Autodesk Inventor part; units mm, degrees
ref_plane "YZ Plane" through (0, 0, 0) normal (1, 0, 0) x (0, 1, 0)
ref_plane "XZ Plane" through (0, 0, 0) normal (0, 1, 0) x (-1, 0, 0)
ref_plane "XY Plane" through (0, 0, 0) normal (0, 0, 1) x (1, 0, 0)
sketch "Sketch1" plane through (0, 0, 0) normal (0, 0, 1) x (1, 0, 0)
  line L0 (-30, 25) -> (30, 25)
  line L1 (30, 25) -> (30, -25)
  line L2 (30, -25) -> (-30, -25)
  line L3 (-30, -25) -> (-30, 25)
  point P0 (0, 0)
  point P1 (30, 0)
  point P2 (0, 25)
  dimension "d0" = 60
  dimension "d1" = 50
extrude "Extrusion1" add sketch "Sketch1" along normal blind 2
fillet "Fillet1" radius 2 4 edges at (30, 25, 1) (-30, 25, 1) (30, -25, 1) (-30, -25, 1)
sketch "Sketch2" plane through (0, 0, 2) normal (0, 0, 1) x (1, 0, 0)
  line L0 (-25, 20) -> (25, 20) construction
  line L1 (25, 20) -> (25, -20) construction
  line L2 (25, -20) -> (-25, -20) construction
  line L3 (-25, -20) -> (-25, 20) construction
  point P0 (0, 0)
  point P1 (25, 0)
  point P2 (0, 20)
  dimension "d5" = 50
  dimension "d6" = 40
hole "Hole1" at (-25, 20, 2) at (25, 20, 2) at (-25, -20, 2) at (25, -20, 2) direction (0, 0, -1) diameter 3.4 end through all
sketch "Sketch3" plane through (0, 0, 2) normal (0, 0, 1) x (1, 0, 0)
  line L0 (-18.5, 19) -> (18.5, 19)
  line L1 (18.5, 19) -> (18.5, -14)
  line L2 (18.5, -14) -> (-18.5, -14)
  line L3 (-18.5, -14) -> (-18.5, 19)
  point P0 (0, 0)
  point P1 (0, 19)
  dimension "d15" = 33
  dimension "d16" = 37
  dimension "d17" = 14
extrude "Extrusion2" cut sketch "Sketch3" against normal blind 2
fillet "Fillet2" radius 2 4 edges at (-18.5, 19, 1) (18.5, 19, 1) (18.5, -14, 1) (-18.5, -14, 1)
sketch "Sketch4" plane through (0, 0, 2) normal (0, 0, 1) x (1, 0, 0)
  line L0 (-6.75, -17.5) -> (14.75, -17.5) construction
  line L1 (16.5, -14) -> (-16.5, -14)
  point P0 (0, 0)
  point P1 (4, -17.5)
  dimension "d21" = 21.5
  dimension "d22" = 3.5
  dimension "d33" = 4
hole "Hole2" at (-6.75, -17.5, 2) at (14.75, -17.5, 2) direction (0, 0, -1) diameter 3.4 end through all
chamfer "Chamfer1" distance 0.4 angle 45 44 edges at (0, 25, 2) (-29.4142, 24.4142, 2) (-30, 0, 2) (-29.4142, -24.4142, 2) (0, -25, 2) (29.4142, -24.4142, 2) (30, 0, 2) (29.4142, 24.4142, 2) (0, 25, 0) (-29.4142, 24.4142, 0) (-30, 0, 0) (-29.4142, -24.4142, 0) (0, -25, 0) (29.4142, -24.4142, 0) (30, 0, 0) (29.4142, 24.4142, 0) (-18.5, 2.5, 0) (-17.9142, -13.4142, 0) (0, -14, 0) (17.9142, -13.4142, 0) (18.5, 2.5, 0) (17.9142, 18.4142, 0) (0, 19, 0) (-17.9142, 18.4142, 0) (0, 19, 2) (17.9142, 18.4142, 2) (18.5, 2.5, 2) (17.9142, -13.4142, 2) (0, -14, 2) (-17.9142, -13.4142, 2) (-18.5, 2.5, 2) (-17.9142, 18.4142, 2) (-25, -18.3, 2) (25, -18.3, 2) (-25, 21.7, 2) (25, 21.7, 2) (-6.75, -15.8, 2) (14.75, -15.8, 2) (-25, -18.3, 0) (25, -18.3, 0) (-25, 21.7, 0) (25, 21.7, 0) (-6.75, -15.8, 0) (14.75, -15.8, 0)
properties part number "bradboardclip" material "ABS Plastic"
Build history of the part. All positions in model axes, mm. A direction names the side the tool comes from. Give positions to 0.01 mm unless a question says otherwise; leave off trailing zeros. Loops run counter-clockwise (first coordinate to the right, second up) from the corner with the lowest first, then second, coordinate; pieces in that order, holes last. Notation, with made-up numbers: (17.25, 33) - (75.25, 33) arc R12 cw to (75.25, 48) - close; hole circle Ø8 at (6, 49). An arc over 180 degrees is marked (long way). Use a Markdown table: item, result.
(1) Wall check: line 1 along X through (y, z) = (20, 1.4); line 2 along Y through (x, z) = (25, 1.05); line 3 along X through (y, z) = (-17.5, 0.85). Give the ranges that are in metal, low to high.
Taken from the geometry:
| item | result |
|---|---|
| line 1 | -30 to -26.7, -23.3 to 23.3, 26.7 to 30 |
| line 2 | -25 to -21.7, -18.3 to 18.3, 21.7 to 25 |
| line 3 | -30 to -8.45, -5.05 to 13.05, 16.45 to 30 |
(2) Band-saw the part on C-C (y = 14). Give the cut face in (x, z), and give its area (3 significant figures).
Taken from the geometry:
| item | result |
|---|---|
| outline | (-30, 0.4) - (-29.6, 0) - (-18.9, 0) - (-18.5, 0.4) - (-18.5, 1.6) - (-18.9, 2) - (-29.6, 2) - (-30, 1.6) - close; (18.5, 0.4) - (18.9, 0) - (29.6, 0) - (30, 0.4) - (30, 1.6) - (29.6, 2) - (18.9, 2) - (18.5, 1.6) - close |
| area | 45.4 mm2 |
(3) Drop flat-ended pins along their axis: pin 1 Ø3 at (x, y) = (-25, -20) entering from -Z; pin 2 Ø4 at (x, y) = (25, -20) entering from +Z; pin 3 Ø4 at (x, y) = (-25, 20) entering from -Z. Give the stop position or say it passes through.
Taken from the geometry:
| item | result |
|---|---|
| pin 1 | through |
| pin 2 | z = 1.9 |
| pin 3 | z = 0.1 |
(4) Band-saw the part on B-B (x = 25). Give the cut face in (y, z), and give its area (3 significant figures).
Taken from the geometry:
| item | result |
|---|---|
| outline | (-25, 0.4) - (-24.6, 0) - (-22.1, 0) - (-21.7, 0.4) - (-21.7, 1.6) - (-22.1, 2) - (-24.6, 2) - (-25, 1.6) - close; (-18.3, 0.4) - (-17.9, 0) - (17.9, 0) - (18.3, 0.4) - (18.3, 1.6) - (17.9, 2) - (-17.9, 2) - (-18.3, 1.6) - close; (21.7, 0.4) - (22.1, 0) - (24.6, 0) - (25, 0.4) - (25, 1.6) - (24.6, 2) - (22.1, 2) - (21.7, 1.6) - close |
| area | 85.4 mm2 |
(5) Pull direction Y, two halves, no side cores. Call faces 1 (the face through (0, -25, 1)), 2 (the face through (30, 0, 1)), 3 (the face through (17.978, 18.511, 0.286)), 4 (the face through (-17.978, 18.511, 1.714)): +Y half, -Y half, draft (parallel to the pull), parting line (faces both ways), or undercut.
Taken from the geometry:
| item | result |
|---|---|
| face 1 | -Y half |
| face 2 | draft |
| face 3 | undercut |
| face 4 | undercut |
(6) Band-saw the part on A-A (x = 1.5). Give the cut face in (y, z).
Taken from the geometry:
| item | result |
|---|---|
| outline | (-25, 0.4) - (-24.6, 0) - (-14.4, 0) - (-14, 0.4) - (-14, 1.6) - (-14.4, 2) - (-24.6, 2) - (-25, 1.6) - close; (19, 0.4) - (19.4, 0) - (24.6, 0) - (25, 0.4) - (25, 1.6) - (24.6, 2) - (19.4, 2) - (19, 1.6) - close |
(7) Band-saw the part on D-D (z = 0.95). Give the cut face in (x, y), and give its area (3 significant figures).
Taken from the geometry:
| item | result |
|---|---|
| outline | (-30, -23) arc R2 ccw to (-28, -25) - (28, -25) arc R2 ccw to (30, -23) - (30, 23) arc R2 ccw to (28, 25) - (-28, 25) arc R2 ccw to (-30, 23) - close; hole circle Ø3.4 at (-25, -20); hole circle Ø3.4 at (-25, 20); hole (-18.5, -12) arc R2 ccw to (-16.5, -14) - (16.5, -14) arc R2 ccw to (18.5, -12) - (18.5, 17) arc R2 ccw to (16.5, 19) - (-16.5, 19) arc R2 ccw to (-18.5, 17) - close; hole circle Ø3.4 at (-6.75, -17.5); hole circle Ø3.4 at (14.75, -17.5); hole circle Ø3.4 at (25, -20); hole circle Ø3.4 at (25, 20) |
| area | 1,720 mm2 |
(8) Which spindle directions (+Z, -Z, +X, -X, +Y, -Y) get a long thin tool onto all of the face, cutting with end or side? Do faces 5 (the face through (0, -14, 1)), 6 (the face through (-18.011, 18.478, 0.286)), 7 (the face through (0, -16, 0)). Say none if no direction does.
Taken from the geometry:
| item | result |
|---|---|
| face 5 | +Z, -Z |
| face 6 | -Z |
| face 7 | -Z, +X, -X, +Y, -Y |
